For this review, take the finished solid that the model builds, in its own axes (mm). Face numbers are marked on the shaded views. A direction names the side the tool comes from. Round coordinates to 2 decimals unless told otherwise and drop trailing zeros. Order: outer loops, then holes, each group sorted by start corner. A loop starts at its lowest first (then second) coordinate and runs counter-clockwise, first axis right, second up. Notation, with made-up numbers: (-10, 12.25) -> (12, 12.25) arc R27 cw to (12, 46.25) -> close; hole circle Ø6 at (6.25, -33). An arc over 180 degrees is marked (long way). Answer in a Markdown table with one row per item.
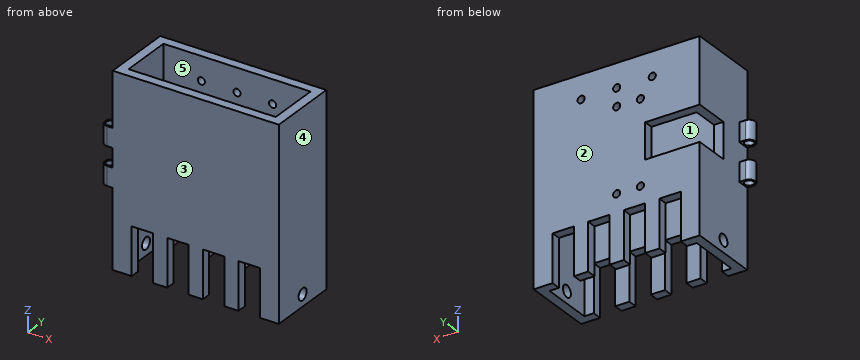
```python
from build123d import *

# Parameters (mm, degrees)
SKETCH1_W               = 88.9
SKETCH1_H               = 101.6
BOSS_EXTRUDE1_DEPTH     = 38.1
SHELL1_T                = -5.08
CUT_EXTRUDE3_START      = -19.05
SKETCH4_W               = 29.21
SKETCH4_H               = 19.05
CUT_EXTRUDE3_DEPTH      = 20.05
SKETCH5_W               = 11.43
SKETCH5_H               = 25.4
CUT_EXTRUDE4_DEPTH      = 39.1
SKETCH6_R               = 3.175
CUT_EXTRUDE5_DEPTH      = 4.2672
CUT_EXTRUDE5_DEPTH_BACK = 89.9
CUT_EXTRUDE6_REACH      = 40.1
SKETCH7_R               = 1.905
SKETCH9_W               = 10.16
SKETCH9_H               = 6.35
BOSS_EXTRUDE2_DEPTH     = 6.35
SKETCH10_R              = 2.38125
CUT_EXTRUDE7_DEPTH      = 30.48


with BuildPart() as part:
    # Sketch1 → Boss-Extrude1 (new body)
    with BuildSketch(Plane(origin=(0, 0, 0), x_dir=(1, 0, 0), z_dir=(0, 1, 0))):
        with Locations((44.45, 50.8)):
            Rectangle(SKETCH1_W, SKETCH1_H)
    extrude(amount=BOSS_EXTRUDE1_DEPTH)

    # Shell1
    shell1_openings = [part.faces().sort_by_distance(p)[0] for p in [
        (44.45, 19.05, 0),
        (44.45, 19.05, -101.6),
    ]]
    offset(amount=SHELL1_T, openings=shell1_openings, kind=Kind.INTERSECTION)

    # Sketch4 → Cut-Extrude3 (cut, through all)
    with BuildSketch(Plane.XZ.offset(CUT_EXTRUDE3_START)):
        with Locations((14.605, -44.45)):
            Rectangle(SKETCH4_W, SKETCH4_H)
    extrude(amount=-CUT_EXTRUDE3_DEPTH, mode=Mode.SUBTRACT)

    # Sketch5 → Cut-Extrude4 (cut, through all)
    with BuildSketch(Plane(origin=(0, 38.1, 0), x_dir=(1, 0, 0), z_dir=(0, 1, 0))):
        with Locations((15.875, 88.9)):
            Rectangle(SKETCH5_W, SKETCH5_H)
        with Locations((34.925, 88.9)):
            Rectangle(SKETCH5_W, SKETCH5_H)
        with Locations((53.975, 88.9)):
            Rectangle(SKETCH5_W, SKETCH5_H)
        with Locations((73.025, 88.9)):
            Rectangle(SKETCH5_W, SKETCH5_H)
    extrude(amount=-CUT_EXTRUDE4_DEPTH, mode=Mode.SUBTRACT)

    # Sketch6 → Cut-Extrude5 (cut, two sides)
    with BuildSketch(Plane.ZY) as cut_extrude5_sk:
        with Locations((-95.25, 19.05)):
            Circle(SKETCH6_R)
    extrude(amount=CUT_EXTRUDE5_DEPTH, mode=Mode.SUBTRACT)
    extrude(cut_extrude5_sk.sketch, amount=-CUT_EXTRUDE5_DEPTH_BACK, mode=Mode.SUBTRACT)

    # Sketch7 → Cut-Extrude6 (cut, up to next)
    with BuildSketch(Plane(origin=(0, 38.1, 0), x_dir=(1, 0, 0), z_dir=(0, 1, 0)), mode=Mode.PRIVATE) as cut_extrude6_sk1:
        with Locations((44.45, 12.7)):
            Circle(SKETCH7_R)
    cut_extrude6_tool1 = extrude(cut_extrude6_sk1.sketch, amount=-CUT_EXTRUDE6_REACH, mode=Mode.PRIVATE) & part.part
    add(cut_extrude6_tool1.solids().sort_by_distance((44.45, 38.1, -12.7))[0], mode=Mode.SUBTRACT)
    # Sketch7 → Cut-Extrude6 (cut, up to next)
    with BuildSketch(Plane(origin=(0, 38.1, 0), x_dir=(1, 0, 0), z_dir=(0, 1, 0)), mode=Mode.PRIVATE) as cut_extrude6_sk2:
        with Locations((25.4, 12.7)):
            Circle(SKETCH7_R)
    cut_extrude6_tool2 = extrude(cut_extrude6_sk2.sketch, amount=-CUT_EXTRUDE6_REACH, mode=Mode.PRIVATE) & part.part
    add(cut_extrude6_tool2.solids().sort_by_distance((25.4, 38.1, -12.7))[0], mode=Mode.SUBTRACT)
    # Sketch7 → Cut-Extrude6 (cut, up to next)
    with BuildSketch(Plane(origin=(0, 38.1, 0), x_dir=(1, 0, 0), z_dir=(0, 1, 0)), mode=Mode.PRIVATE) as cut_extrude6_sk3:
        with Locations((63.5, 12.7)):
            Circle(SKETCH7_R)
    cut_extrude6_tool3 = extrude(cut_extrude6_sk3.sketch, amount=-CUT_EXTRUDE6_REACH, mode=Mode.PRIVATE) & part.part
    add(cut_extrude6_tool3.solids().sort_by_distance((63.5, 38.1, -12.7))[0], mode=Mode.SUBTRACT)
    # Sketch7 → Cut-Extrude6 (cut, up to next)
    with BuildSketch(Plane(origin=(0, 38.1, 0), x_dir=(1, 0, 0), z_dir=(0, 1, 0)), mode=Mode.PRIVATE) as cut_extrude6_sk4:
        with Locations((31.75, 66.675)):
            Circle(SKETCH7_R)
    cut_extrude6_tool4 = extrude(cut_extrude6_sk4.sketch, amount=-CUT_EXTRUDE6_REACH, mode=Mode.PRIVATE) & part.part
    add(cut_extrude6_tool4.solids().sort_by_distance((31.75, 38.1, -66.675))[0], mode=Mode.SUBTRACT)
    # Sketch7 → Cut-Extrude6 (cut, up to next)
    with BuildSketch(Plane(origin=(0, 38.1, 0), x_dir=(1, 0, 0), z_dir=(0, 1, 0)), mode=Mode.PRIVATE) as cut_extrude6_sk5:
        with Locations((44.45, 66.675)):
            Circle(SKETCH7_R)
    cut_extrude6_tool5 = extrude(cut_extrude6_sk5.sketch, amount=-CUT_EXTRUDE6_REACH, mode=Mode.PRIVATE) & part.part
    add(cut_extrude6_tool5.solids().sort_by_distance((44.45, 38.1, -66.675))[0], mode=Mode.SUBTRACT)
    # Sketch7 → Cut-Extrude6 (cut, up to next)
    with BuildSketch(Plane(origin=(0, 38.1, 0), x_dir=(1, 0, 0), z_dir=(0, 1, 0)), mode=Mode.PRIVATE) as cut_extrude6_sk6:
        with Locations((44.45, 22.225)):
            Circle(SKETCH7_R)
    cut_extrude6_tool6 = extrude(cut_extrude6_sk6.sketch, amount=-CUT_EXTRUDE6_REACH, mode=Mode.PRIVATE) & part.part
    add(cut_extrude6_tool6.solids().sort_by_distance((44.45, 38.1, -22.225))[0], mode=Mode.SUBTRACT)
    # Sketch7 → Cut-Extrude6 (cut, up to next)
    with BuildSketch(Plane(origin=(0, 38.1, 0), x_dir=(1, 0, 0), z_dir=(0, 1, 0)), mode=Mode.PRIVATE) as cut_extrude6_sk7:
        with Locations((31.75, 22.225)):
            Circle(SKETCH7_R)
    cut_extrude6_tool7 = extrude(cut_extrude6_sk7.sketch, amount=-CUT_EXTRUDE6_REACH, mode=Mode.PRIVATE) & part.part
    add(cut_extrude6_tool7.solids().sort_by_distance((31.75, 38.1, -22.225))[0], mode=Mode.SUBTRACT)

    # Sketch9 → Boss-Extrude2 (add)
    with BuildSketch(Plane.ZY):
        with Locations((-34.29, 3.175)):
            Rectangle(SKETCH9_W, SKETCH9_H)
        with Locations((-54.61, 3.175)):
            Rectangle(SKETCH9_W, SKETCH9_H)
    extrude(amount=BOSS_EXTRUDE2_DEPTH)

    # Sketch10 → Cut-Extrude7 (cut)
    with BuildSketch(Plane.XY.offset(-29.21)):
        with Locations((-3.175, 3.175)):
            Circle(SKETCH10_R)
        with BuildLine():
            Line((-3.175, 7.665128061), (-3.175, 6.35))
            ThreePointArc((-3.175, 6.35), (-6.35, 3.175), (-3.175, 0))
            Line((-3.175, 0), (-3.175, -1.315128061))
            ThreePointArc((-3.175, -1.315128061), (-7.665128061, 3.175), (-3.175, 7.665128061))
        make_face()
    extrude(amount=-CUT_EXTRUDE7_DEPTH, mode=Mode.SUBTRACT)


solid = part.part
```
Q1. Tool access review of the marked faces 1 and 2: name each direction out of +Z, -Z, +X, -X, +Y, -Y from which nothing blocks a thin tool from reaching the whole face with its end or side.
Answer key:
| item | result |
|---|---|
| face 1 | +Z, -Z |
| face 2 | +Z, -Z, +X, -X, +Y |
Q2. Clearance check with flat-ended pins moving along their axes: pin 1 Ø1.5 at (y, z) = (35.5, -92.5) entering from -X; pin 2 Ø1.9 at (x, y) = (-2, 4.5) entering from +Z; pin 3 Ø5.5 at (x, y) = (36.5, 3) entering from -Z. State where each tip first meets the part, or that it passes through.
Answer key:
| item | result |
|---|---|
| pin 1 | stops at x = 0 |
| pin 2 | stops at z = -29.21 |
| pin 3 | stops at z = -76.2 |
Q3. To check wall thickness, follow probe 1 along Z at (x, y) = (44.45, 34.9) (3 decimals); probe 2 along X at (y, z) = (36.2, -12.7) (3 decimals); probe 3 along Z at (x, y) = (3, 34) (3 decimals). State the ranges of each line that lie inside material, in increasing order.
Answer key:
| item | result |
|---|---|
| probe 1 | z = -101.6 to -68.58, -64.77 to -24.13, -20.32 to -14.605, -10.795 to 0 |
| probe 2 | x = 0 to 23.495, 27.305 to 42.545, 46.355 to 61.595, 65.405 to 88.9 |
| probe 3 | z = -101.6 to -53.975, -34.925 to 0 |
Q4. The part is to be moulded in two halves that separate along X. For the marked faces 3, 4 and 5, say which applies: +X half, -X half, draft (parallel to the pull), parting line (faces both ways), or undercut.
Answer key:
| item | result |
|---|---|
| face 3 | draft |
| face 4 | +X half |
| face 5 | undercut |
Q5. Take a section at D-D, the plane y = 14. Write out the cut boundary in (x, z), then the cut area to 3 significant figures.
Answer key:
| item | result |
|---|---|
| outline | (0, -101.6) -> (5.08, -101.6) -> (5.08, 0) -> (0, 0) -> close; (83.82, -101.6) -> (88.9, -101.6) -> (88.9, 0) -> (83.82, 0) -> close |
| area | 1,030 mm^2 |
Q6. Take a section at C-C, the plane x = 25.4. Write out the cut boundary in (y, z) (3 decimals).
Answer key:
| item | result |
|---|---|
| outline | (0, -101.6) -> (5.08, -101.6) -> (5.08, 0) -> (0, 0) -> close; (33.02, -101.6) -> (38.1, -101.6) -> (38.1, -53.975) -> (33.02, -53.975) -> close; (33.02, -34.925) -> (38.1, -34.925) -> (38.1, -14.605) -> (33.02, -14.605) -> close; (33.02, -10.795) -> (38.1, -10.795) -> (38.1, 0) -> (33.02, 0) -> close |
Q7. Take a section at B-B, the plane z = -12.7. Write out the cut boundary in (x, y) (3 decimals).
Answer key:
| item | result |
|---|---|
| outline | (0, 0) -> (88.9, 0) -> (88.9, 38.1) -> (65.405, 38.1) -> (65.405, 33.02) -> (83.82, 33.02) -> (83.82, 5.08) -> (5.08, 5.08) -> (5.08, 33.02) -> (23.495, 33.02) -> (23.495, 38.1) -> (0, 38.1) -> close; (27.305, 33.02) -> (42.545, 33.02) -> (42.545, 38.1) -> (27.305, 38.1) -> close; (46.355, 33.02) -> (61.595, 33.02) -> (61.595, 38.1) -> (46.355, 38.1) -> close |
Q8. Take a section at A-A, the plane x = 54.5. Write out the cut boundary in (y, z).
Answer key:
| item | result |
|---|---|
| outline | (0, -76.2) -> (5.08, -76.2) -> (5.08, 0) -> (0, 0) -> close; (33.02, -76.2) -> (38.1, -76.2) -> (38.1, 0) -> (33.02, 0) -> close |
